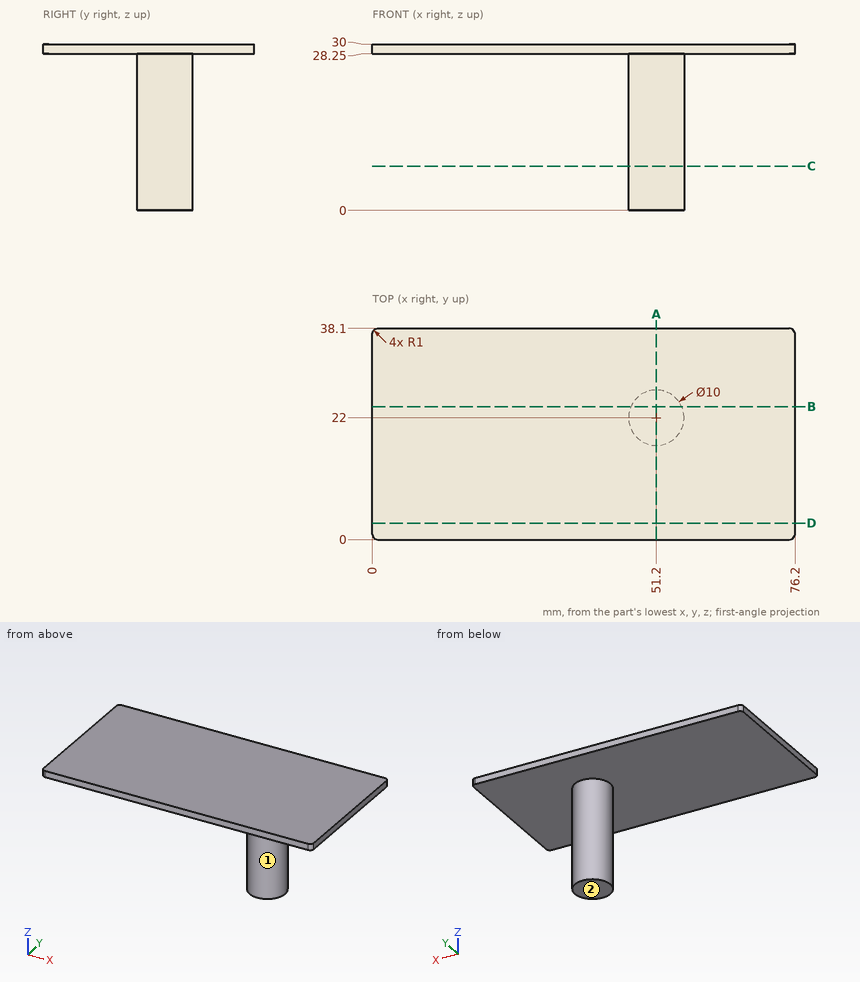
Geometry check sheet. Reference: drawing and pictorial views, mm from the part's lowest x, y, z. A direction names the side the tool comes from. Round coordinates to 2 decimals unless told otherwise and drop trailing zeros. Write each loop counter-clockwise with the first axis right and the second up, starting at its lowest first coordinate (ties: lowest second). Pieces come first, ordered by that corner, then holes.
Item 1: Section check A-A (x = 51.2). Record the boundary of the cut face in (y, z).
Determined:
outline: (0, 28.25) - (17, 28.25) - (17, 0) - (27, 0) - (27, 28.25) - (38.1, 28.25) - (38.1, 30) - (0, 30) - close
Item 2: Material ranges on line 1 along Z through (x, y) = (14, 32); line 2 along Y through (x, z) = (52, 14); line 3 along Y through (x, z) = (55, 10.75), recorded low to high.
Determined:
line 1: z = 28.25 to 30
line 2: y = 17.06 to 26.94
line 3: y = 18.75 to 25.25
Item 3: Section check D-D (y = 3). Record the boundary of the cut face in (x, z).
Determined:
outline: (0, 28.25) - (76.2, 28.25) - (76.2, 30) - (0, 30) - close
Item 4: Go/stop test with flat-tipped pins: pin 1 Ø6 at (x, z) = (47, 20) entering from +Y; pin 2 Ø8 at (y, z) = (30, 3.5) entering from -X. Record where each tip stops, or that it passes through.
Determined:
pin 1: stops at y = 26.85
pin 2: stops at x = 48.2
Item 5: Section check B-B (y = 24). Record the boundary of the cut face in (x, z).
Determined:
outline: (0, 28.25) - (46.62, 28.25) - (46.62, 0) - (55.78, 0) - (55.78, 28.25) - (76.2, 28.25) - (76.2, 30) - (0, 30) - close
Item 6: Access from +Z, -Z, +X, -X, +Y, -Y to the whole of each face (thin tool, end or side, straight path). Record for the marked faces 1 and 2.
Determined:
face 1: -Z
face 2: -Z, +X, -X, +Y, -Y
Item 7: Section check C-C (z = 8). Record the boundary of the cut face in (x, y), plus the area to 3 significant figures.
Determined:
outline: circle Ø10 at (51.2, 22)
area: 78.5 mm2
